Source: CAD feature listing. Evaluate the final solid. Frame: model axes, mm. Face numbers are marked on the shaded views. A direction names the side the tool comes from. Give positions to 0.01 mm unless a question says otherwise; leave off trailing zeros. Loops run counter-clockwise (first coordinate to the right, second up) from the corner with the lowest first, then second, coordinate; pieces in that order, holes last. Notation, with made-up numbers: M -21.75,-15 L 33.25,-15 A14 cw 33.25,1 Z; hole C -40,-8 d11. An arc over 180 degrees is marked long. Answer in a Markdown table with one row per item.
```python
from build123d import *

# Parameters (mm, degrees)
SKETCH_W          = 45
SKETCH_H          = 29
PAD_DEPTH         = 45
SKETCH001_W       = 40
SKETCH001_H       = 24
POCKET_DEPTH      = 0.001
POCKET_DEPTH_BACK = 45.001
SKETCH002_R       = 3.62
POCKET001_DEPTH   = 3.5
SKETCH003_R       = 2
POCKET002_DEPTH   = 2.5
CHAMFER_SIZE      = 2.485
SKETCH004_W       = 45
SKETCH004_H       = 29
PAD001_DEPTH      = 2
FILLET_R          = 1


with BuildPart() as part:
    # Sketch → Pad (new body)
    with BuildSketch(Plane.XZ):
        Rectangle(SKETCH_W, SKETCH_H)
    extrude(amount=PAD_DEPTH)

    # Sketch001 → Pocket (cut, two sides)
    with BuildSketch(Plane.XZ) as pocket_sk:
        Rectangle(SKETCH001_W, SKETCH001_H)
    extrude(amount=-POCKET_DEPTH, mode=Mode.SUBTRACT)
    extrude(pocket_sk.sketch, amount=POCKET_DEPTH_BACK, mode=Mode.SUBTRACT)

    # Sketch002 (on DatumPlane) → Pocket001 (cut)
    with BuildSketch(Plane(origin=(0, 0, 14.5), x_dir=(-1, 0, 0), z_dir=(0, 0, 1))):
        with Locations((-10.625, 22.5)):
            Circle(SKETCH002_R)
        with Locations((10.625, 22.5)):
            Circle(SKETCH002_R)
    extrude(amount=-POCKET001_DEPTH, mode=Mode.SUBTRACT)

    # Sketch003 (on DatumPlane) → Pocket002 (cut)
    with BuildSketch(Plane(origin=(0, 0, -12), x_dir=(-1, 0, 0), z_dir=(0, 0, 1))):
        with Locations((-10.625, 22.5)):
            Circle(SKETCH003_R)
        with Locations((10.625, 22.5)):
            Circle(SKETCH003_R)
    extrude(amount=-POCKET002_DEPTH, mode=Mode.SUBTRACT)

    # Chamfer
    chamfer_edges = [part.edges().sort_by_distance(p)[0] for p in [
        (-8.625, -22.5, -12),
        (12.625, -22.5, -12),
    ]]
    chamfer(chamfer_edges, length=CHAMFER_SIZE)

    # Sketch004 → Pad001 (join)
    with BuildSketch(Plane.XZ):
        Rectangle(SKETCH004_W, SKETCH004_H)
    extrude(amount=PAD001_DEPTH)

    # Fillet
    fillet_edges = [part.edges().sort_by_distance(p)[0] for p in [
        (-22.5, -45, 0),
        (0, -45, 14.5),
        (0, -45, -14.5),
        (22.5, -45, 0),
        (-20, -45, 0),
        (0, -45, 12),
        (20, -45, 0),
        (0, -45, -12),
        (22.5, -23.5, 14.5),
        (22.5, -23.5, -14.5),
        (-22.5, -23.5, 14.5),
        (-22.5, -23.5, -14.5),
        (0, 0, 14.5),
        (-22.5, 0, 0),
        (22.5, 0, 0),
        (22.5, -1, 14.5),
        (-22.5, -1, 14.5),
        (-22.5, -1, -14.5),
        (22.5, -1, -14.5),
        (0, 0, -14.5),
        (-7.005, -22.5, 14.5),
        (14.245, -22.5, 14.5),
    ]]
    fillet(fillet_edges, radius=FILLET_R)


solid = part.part
```
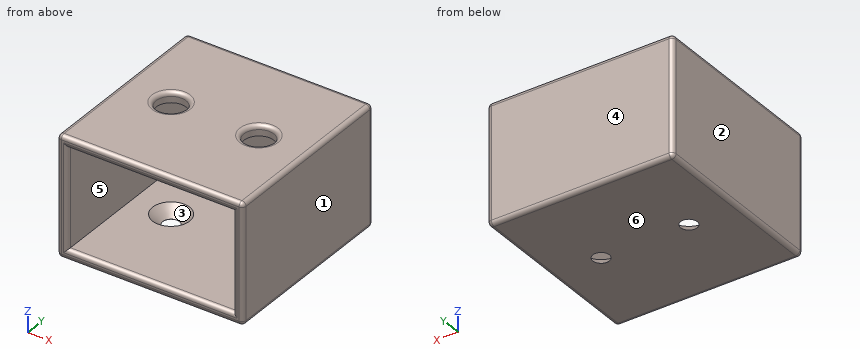
Q1. Mould query, pull axis X, two halves, no side actions, for the marked faces 1, 2, 3 and 4. Classes: +X half, -X half, draft (parallel to the pull), parting line (faces both ways), or undercut.
Values follow:
| item | result |
|---|---|
| face 1 | +X half |
| face 2 | -X half |
| face 3 | undercut |
| face 4 | draft |
Q2. Reachability of the marked faces 5 and 6 from +Z, -Z, +X, -X, +Y, -Y: full face, straight path, thin tool, end or side. Return the list, or none.
Values follow:
| item | result |
|---|---|
| face 5 | -Y |
| face 6 | -Z, +X, -X, +Y, -Y |
Q3. Contact query for flat-ended pins moving along their axis: pin 1 Ø4.5 at (x, y) = (10.625, -22.5) entering from +Z (3 decimals); pin 2 Ø1.5 at (x, z) = (-11, -0.5) entering from -Y; pin 3 Ø8.5 at (x, y) = (-10.625, -22.5) entering from +Z. Output: stop coordinate, or through.
Values follow:
| item | result |
|---|---|
| pin 1 | z = -14.235 |
| pin 2 | y = -2 |
| pin 3 | z = 14.43 |
Q4. Section query B-B (x = -19). Output: boundary loops of the cut face in (y, z), plus the area to 3 significant figures.
Values follow:
| item | result |
|---|---|
| outline | M -45,-13.5 A1 ccw -44,-14.5 L -1,-14.5 A1 ccw 0,-13.5 L 0,13.5 A1 ccw -1,14.5 L -44,14.5 A1 ccw -45,13.5 L -45,13 A1 ccw -44,12 L -2,12 L -2,-12 L -44,-12 A1 ccw -45,-13 Z |
| area | 272 mm^2 |
Q5. Section query C-C (z = -10). Output: boundary loops of the cut face in (x, y).
Values follow:
| item | result |
|---|---|
| outline | M -22.5,-44 A1 ccw -21.5,-45 L -21,-45 A1 ccw -20,-44 L -20,-2 L 20,-2 L 20,-44 A1 ccw 21,-45 L 21.5,-45 A1 ccw 22.5,-44 L 22.5,-1 A1 ccw 21.5,0 L -21.5,0 A1 ccw -22.5,-1 Z |
Q6. Section query D-D (y = -22.5). Give the number of separate pieces and of enclosed holes in the cut face, plus the area to 3 significant figures.
Values follow:
| item | result |
|---|---|
| separate pieces | 4 |
| enclosed holes | 0 |
| area | 275 mm^2 |
Q7. Ray query, probe 1 along X at (y, z) = (-22.5, 13) (3 decimals); probe 2 along Z at (x, y) = (-16.5, -14); probe 3 along X at (y, z) = (-39, 4.5). Return the intervals inside material, ascending. Write a range as from..to.
Values follow:
| item | result |
|---|---|
| probe 1 | -22.5..-14.245, -7.005..7.005, 14.245..22.5 |
| probe 2 | -14.5..-12, 12..14.5 |
| probe 3 | -22.5..-20, 20..22.5 |
Q8. Section query A-A (y = -7). Output: boundary loops of the cut face in (x, z), plus the area to 3 significant figures.
Values follow:
| item | result |
|---|---|
| outline | M -22.5,-13.5 A1 ccw -21.5,-14.5 L 21.5,-14.5 A1 ccw 22.5,-13.5 L 22.5,13.5 A1 ccw 21.5,14.5 L -21.5,14.5 A1 ccw -22.5,13.5 Z; hole M -20,-12 L 20,-12 L 20,12 L -20,12 Z |
| area | 344 mm^2 |
